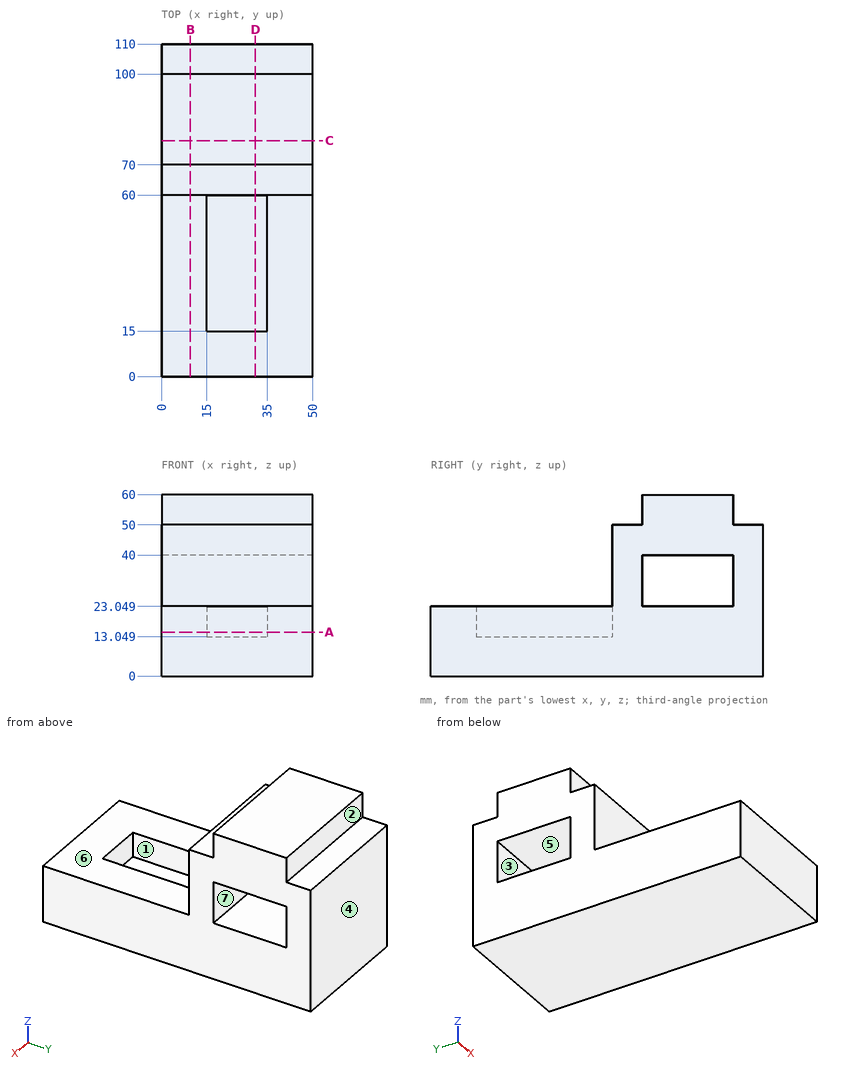
Source: three-view drawing plus pictorial views. Frame: mm from the lowest corner of the part. A direction names the side the tool comes from. Round coordinates to 2 decimals unless told otherwise and drop trailing zeros. Loops run counter-clockwise (first coordinate to the right, second up) from the corner with the lowest first, then second, coordinate; pieces in that order, holes last.
Q1. Pull-direction query (Y, two-part tool) for the marked faces 4, 5, 6 and 7; classes: released by +Y, released by -Y, zero draft, split by the parting line, or undercut.
Q2. Section C-C on y = 78. Return loops of the section in (x, z).
Q3. Material intervals for L1, parallel to Y at x = 8.5, z = 24.5; L2, parallel to X at y = 30, z = 16; L3, parallel to Y at x = 17.5, z = 23, sorted ascending.
Q4. Section A-A on z = 14.5. Return loops of the section in (x, y), plus the area to 3 significant figures.
Q5. Section D-D on x = 31. Return loops of the section in (y, z).
Q6. Access query for the marked faces 1, 2 and 3. Directions: +Z, -Z, +X, -X, +Y, -Y. A direction counts if a zero-diameter tool reaches every point of the face in a straight line with its end or side. Return the directions, or none.
Q7. Section B-B on x = 9.5. Return loops of the section in (y, z).
Q8. Pin query (flat end, axial travel): P1, Ø8, axis at x = 33.5, z = 55, coming from the +Y side; P2, Ø11, axis at x = 13.5, z = 52.5, coming from the -Y side; P3, Ø3, axis at x = 26, y = 106.5, coming from the +Z side. Return the tip coordinate at first contact, or that it passes through.
Evaluation:
1. face 4: released by +Y
1. face 5: undercut
1. face 6: zero draft
1. face 7: undercut
2. outline: (0, 0) - (50, 0) - (50, 23.05) - (0, 23.05) - close; (0, 40) - (50, 40) - (50, 60) - (0, 60) - close
3. L1: y = 60 to 70, 100 to 110
3. L2: x = 0 to 15, 35 to 50
3. L3: y = 0 to 15, 60 to 110
4. outline: (0, 0) - (50, 0) - (50, 110) - (0, 110) - close; hole (15, 15) - (35, 15) - (35, 60) - (15, 60) - close
4. area: 4,600 mm2
5. outline: (0, 0) - (110, 0) - (110, 50) - (100, 50) - (100, 60) - (70, 60) - (70, 50) - (60, 50) - (60, 13.05) - (15, 13.05) - (15, 23.05) - (0, 23.05) - close; hole (70, 23.05) - (100, 23.05) - (100, 40) - (70, 40) - close
6. face 1: +Z
6. face 2: +Z, +X, -X, +Y
6. face 3: +X, -X
7. outline: (0, 0) - (110, 0) - (110, 50) - (100, 50) - (100, 60) - (70, 60) - (70, 50) - (60, 50) - (60, 23.05) - (0, 23.05) - close; hole (70, 23.05) - (100, 23.05) - (100, 40) - (70, 40) - close
8. P1: stops at y = 100
8. P2: stops at y = 60
8. P3: stops at z = 50
